Read the model definition and answer for the solid it produces. Units are mm, in the model's axes. Give positions to 0.01 mm unless a question says otherwise; leave off trailing zeros. Write each loop counter-clockwise with the first axis right and the second up, starting at its lowest first coordinate (ties: lowest second). Pieces come first, ordered by that corner, then holes.
```python
from build123d import *

# Parameters (mm, degrees)
SKETCH1_W           = 20
SKETCH1_H           = 20
BOSS_EXTRUDE1_DEPTH = 2.5
SKETCH2_R           = 0.5
CUT_EXTRUDE1_DEPTH  = 21
SKETCH3_R           = 2
CUT_EXTRUDE2_DEPTH  = 3.5


with BuildPart() as part:
    # Sketch1 → Boss-Extrude1 (new body)
    with BuildSketch(Plane(origin=(0, 0, 0), x_dir=(1, 0, 0), z_dir=(0, 1, 0))):
        with Locations((-50.754716981, 42.075471698)):
            Rectangle(SKETCH1_W, SKETCH1_H)
    extrude(amount=BOSS_EXTRUDE1_DEPTH)

    # Sketch2 → Cut-Extrude1 (cut, through all)
    with BuildSketch(Plane.XY.offset(-32.075471698)):
        with Locations((-50.754716981, 2.75)):
            Circle(SKETCH2_R)
    extrude(amount=-CUT_EXTRUDE1_DEPTH, mode=Mode.SUBTRACT)

    # Sketch3 → Cut-Extrude2 (cut, through all)
    with BuildSketch(Plane(origin=(0, 2.5, 0), x_dir=(1, 0, 0), z_dir=(0, 1, 0))):
        with Locations((-55.754716981, 42.075471698)):
            Circle(SKETCH3_R)
        with Locations((-45.754716981, 42.075471698)):
            Circle(SKETCH3_R)
    extrude(amount=-CUT_EXTRUDE2_DEPTH, mode=Mode.SUBTRACT)


solid = part.part
```
Item 1: Determine the mould class of faces 1 (the cylindrical face through (-50.76, 2.25, -41.94)), 2 (the cylindrical face through (-57.342, 1.268, -40.859)), 3 (the flat face through (-51, 1, -32.075)) for opening direction Z: pulls with the +Z half, pulls with the -Z half, needs draft (parallel to the pull), parting line crosses it, or undercut.
Result set:
face 1: needs draft
face 2: undercut
face 3: pulls with the +Z half
Item 2: This flat-tipped pin is pushed along its axis until it touches: pin 1 Ø3.5 at (x, z) = (-55.75, -42.08) entering from +Y. Where does it stop, or does it pass through?
Result set:
pin 1: passes through
Item 3: Section B-B (x = -55.25) is taken. Write down the section's boundary in (y, z).
Result set:
outline: (0, -52.08) - (2.5, -52.08) - (2.5, -44.01) - (0, -44.01) - close; (0, -40.14) - (2.5, -40.14) - (2.5, -32.08) - (0, -32.08) - close
Item 4: Find the intervals of material crossed by line 1 along Z through (x, y) = (-55.75, 0.85); line 2 along Z through (x, y) = (-56.5, 0.1); line 3 along X through (y, z) = (2.45, -39.5), in increasing order.
Result set:
line 1: z = -52.08 to -44.08, -40.08 to -32.08
line 2: z = -52.08 to -43.93, -40.22 to -32.08
line 3: x = -60.75 to -51.15, -50.35 to -40.75
Item 5: Section D-D (z = -43.5) is taken. Write down the section's boundary in (x, y).
Result set:
outline: (-60.75, 0) - (-57.16, 0) - (-57.16, 2.5) - (-60.75, 2.5) - close; (-54.35, 0) - (-47.16, 0) - (-47.16, 2.5) - (-50.32, 2.5) arc R0.5 cw to (-51.19, 2.5) - (-54.35, 2.5) - close; (-44.35, 0) - (-40.75, 0) - (-40.75, 2.5) - (-44.35, 2.5) - close
Item 6: Section C-C (y = 1.15) is taken. Write down the section's boundary in (x, z).
Result set:
outline: (-60.75, -52.08) - (-40.75, -52.08) - (-40.75, -32.08) - (-60.75, -32.08) - close; hole circle Ø4 at (-55.75, -42.08); hole circle Ø4 at (-45.75, -42.08)
Item 7: Section A-A (z = -41.5) is taken. Write down the section's boundary in (x, y).
Result set:
outline: (-60.75, 0) - (-57.67, 0) - (-57.67, 2.5) - (-60.75, 2.5) - close; (-53.84, 0) - (-47.67, 0) - (-47.67, 2.5) - (-50.32, 2.5) arc R0.5 cw to (-51.19, 2.5) - (-53.84, 2.5) - close; (-43.84, 0) - (-40.75, 0) - (-40.75, 2.5) - (-43.84, 2.5) - close
